Design review of the part built by this model. Coordinates are the model's own, in mm. Face numbers are marked on the shaded views. A direction names the side the tool comes from. Give positions to 0.01 mm unless a question says otherwise; leave off trailing zeros. Loops run counter-clockwise (first coordinate to the right, second up) from the corner with the lowest first, then second, coordinate; pieces in that order, holes last. Notation, with made-up numbers: M 79.25,-33 L 89.25,-33 A27 ccw 89.25,-8 Z; hole C 67,19 d10. An arc over 180 degrees is marked long. Use CSV: the item, a comma, the result in double quotes.
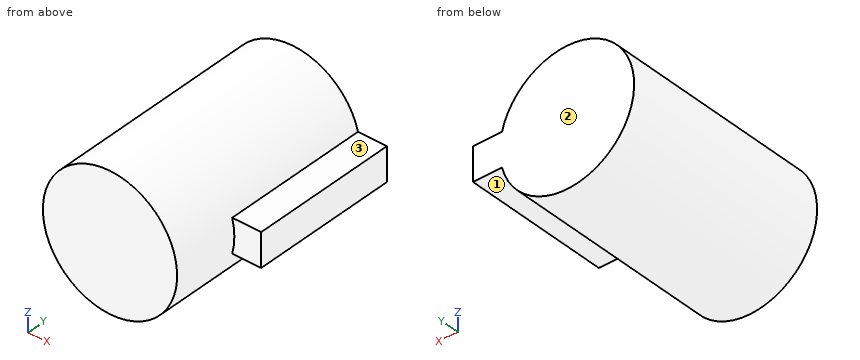
from build123d import *

# Parameters (mm, degrees)
SKETCH1_R           = 5
BOSS_EXTRUDE1_DEPTH = 8
SKETCH2_W           = 7
SKETCH2_H           = 2.5
BOSS_EXTRUDE2_DEPTH = 11


with BuildPart() as part:
    # Sketch1 → Boss-Extrude1 (new, symmetric)
    with BuildSketch(Plane(origin=(0, 0, 0), x_dir=(1, 0, 0), z_dir=(0, 1, 0))):
        with Locations(Location((0, 0, 0), (0, 0, 270))):
            Circle(SKETCH1_R)
    extrude(amount=BOSS_EXTRUDE1_DEPTH, both=True)

    # Sketch2 → Boss-Extrude2 (add)
    with BuildSketch(Plane(origin=(0, 8, 0), x_dir=(1, 0, 0), z_dir=(0, 1, 0))):
        with Locations((3.5, 0)):
            Rectangle(SKETCH2_W, SKETCH2_H)
    extrude(amount=-BOSS_EXTRUDE2_DEPTH)


solid = part.part
(1) We need section A-A on z = 0. State the section outline as (x, y) points, then the cut area to 3 significant figures.
A:
outline,"M -5,-8 L 5,-8 L 5,-3 L 7,-3 L 7,8 L -5,8 Z"
area,"182 mm²"
(2) Wall thickness on line 1 along Y through (x, z) = (5.25, 0); line 2 along X through (y, z) = (2.5, -2.5); line 3 along X through (y, z) = (-2.5, -4.5): over which ranges is each line inside the solid? List them lowest first. Write a range as [from, to].
A:
line 1,"[-3, 8]"
line 2,"[-4.33, 4.33]"
line 3,"[-2.18, 2.18]"
(3) Clearance check with flat-ended pins moving along their axes: P1, Ø1.7, axis at x = 6, y = 2.5, coming from the +Z side; P2, Ø2.5, axis at x = 6.5, y = 1, coming from the -Z side; P3, Ø0.6, axis at x = 6, z = 0.5, coming from the -Y side. State where each tip first meets the part, or that it passes through.
A:
P1,"z = 1.25"
P2,"z = -1.25"
P3,"y = -3"
(4) We need section D-D on y = -1. State the section outline as (x, z) points.
A:
outline,"M 4.84,-1.25 L 7,-1.25 L 7,1.25 L 4.84,1.25 A5 ccw long Z"
(5) We need section B-B on y = -4. State the section outline as (x, z) points.
A:
outline,"C 0,0 d10"
(6) We need section C-C on x = 2. State the section outline as (y, z) points, then the cut area to 3 significant figures.
A:
outline,"M -8,-4.58 L 8,-4.58 L 8,4.58 L -8,4.58 Z"
area,"147 mm²"
(7) Machinability: for the marked faces 1, 2 and 3, which of the approach directions +Z, -Z, +X, -X, +Y, -Y give a long, thin tool a straight path to every point of the face, cutting with its end or side? Answer none if there is none.
A:
face 1,"-Z, +X, +Y, -Y"
face 2,"+Z, -Z, +X, -X, +Y"
face 3,"+Z, +X, +Y, -Y"
